```python
from build123d import *

# Parameters (mm, degrees)
F0_W     = 38.1
F0_H     = 38.1
F1_DEPTH = 76.2
F2_W     = 30.480002
F2_H     = 30.480002
F3_DEPTH = 88.9
F4_W     = 38.1
F4_H     = 31.786919
F5_DEPTH = 3.81


with BuildPart() as f1:
    # F0 (on Top) → F1 (new body)
    with BuildSketch(Plane.XY):
        with Locations((19.05, 19.05)):
            Rectangle(F0_W, F0_H)
    extrude(amount=F1_DEPTH)

    # F2 (on face) → F3 (cut)
    with BuildSketch(Plane.XY.offset(76.2)):
        with Locations((19.05, 19.05)):
            Rectangle(F2_W, F2_H)
    extrude(amount=-F3_DEPTH, mode=Mode.SUBTRACT)

    # F4 (on face) → F5 (cut)
    with BuildSketch(Plane(origin=(0, 38.1, 0), x_dir=(-1, 0, 0), z_dir=(0, 1, 0))):
        with Locations((-19.05, 15.893459)):
            Rectangle(F4_W, F4_H)
    extrude(amount=-F5_DEPTH, mode=Mode.SUBTRACT)


solid = f1.part
```
Work out the finished part from the listing and answer in its coordinate system (mm). A direction names the side the tool comes from. Round coordinates to 2 decimals unless told otherwise and drop trailing zeros. Write each loop counter-clockwise with the first axis right and the second up, starting at its lowest first coordinate (ties: lowest second). Pieces come first, ordered by that corner, then holes. Notation, with made-up numbers: (58, 74) - (63, 74) arc R21 ccw to (63, 81) - close; hole circle Ø1 at (64, 41.5). An arc over 180 degrees is marked (long way). Return JSON: item names as keys, results as strings. Group by question number.
Q1. The part is cut by section C-C on x = 25.5. Write down the section's boundary in (y, z), then the cut area to 3 significant figures.
Q2. For faces 5 (the flat face through (19, 34.29, 54)), 6 (the flat face through (36, 34.29, 16)), 7 (the flat face through (38.1, 19, 38)), determine the directions among +Z, -Z, +X, -X, +Y, -Y from which every point of the face is accessible in a straight line to the end or side of a thin tool.
Q3. The part is cut by section B-B on y = 23. Write down the section's boundary in (x, z).
Q4. The mould has two halves that part along Y. Classify faces 1 (the flat face through (19, 0, 38)), 2 (the flat face through (34.29, 19, 39)), 3 (the flat face through (36, 19, 76.2)), 4 (the flat face through (19, 3.81, 39)): released by +Y, released by -Y, zero draft, split by the parting line, or undercut.
Q5. The part is cut by section D-D on z = 8. Write down the section's boundary in (x, y).
Q6. Find the intervals of material crossed by L1, parallel to Y at x = 23, z = 48; L2, parallel to Y at x = 27, z = 27, in increasing order.
Q7. Each of these flat-tipped pins is pushed along its axis until it touches: pin 1 Ø1.9 at (x, y) = (20, 35.5) entering from -Z; pin 2 Ø1.9 at (x, z) = (35.5, 18.5) entering from +Y; pin 3 Ø3 at (x, z) = (13, 19) entering from +Y. Where does it stop, or does it pass through?
Q8. The part is cut by section A-A on z = 45. Write down the section's boundary in (x, y), then the cut area to 3 significant figures.
Solved:
{
 "1": {"outline": "(0, 0) - (3.81, 0) - (3.81, 76.2) - (0, 76.2) - close; (34.29, 31.79) - (38.1, 31.79) - (38.1, 76.2) - (34.29, 76.2) - close", "area": "460 mm²"},
 "2": {"face 5": "+Z, -Z", "face 6": "-Z, +X, -X, +Y", "face 7": "+Z, -Z, +X, +Y, -Y"},
 "3": {"outline": "(0, 0) - (3.81, 0) - (3.81, 76.2) - (0, 76.2) - close; (34.29, 0) - (38.1, 0) - (38.1, 76.2) - (34.29, 76.2) - close"},
 "4": {"face 1": "released by -Y", "face 2": "undercut", "face 3": "zero draft", "face 4": "undercut"},
 "5": {"outline": "(0, 0) - (38.1, 0) - (38.1, 34.29) - (34.29, 34.29) - (34.29, 3.81) - (3.81, 3.81) - (3.81, 34.29) - (0, 34.29) - close"},
 "6": {"L1": "0 to 3.81, 34.29 to 38.1", "L2": "0 to 3.81"},
 "7": {"pin 1": "z = 31.79", "pin 2": "y = 34.29", "pin 3": "y = 3.81"},
 "8": {"outline": "(0, 0) - (38.1, 0) - (38.1, 38.1) - (0, 38.1) - close; hole (3.81, 3.81) - (34.29, 3.81) - (34.29, 34.29) - (3.81, 34.29) - close", "area": "523 mm²"}
}
